Verification items for this drawing (mm, ordinates from the low corner). Give positions to 0.01 mm unless a question says otherwise; leave off trailing zeros. Write each loop counter-clockwise with the first axis right and the second up, starting at its lowest first coordinate (ties: lowest second). Pieces come first, ordered by that corner, then holes. Notation, with made-up numbers: (48.5, 36) -> (69.5, 36) arc R6 ccw to (69.5, 43) -> close; hole circle Ø5 at (28.25, 74.5). An arc over 180 degrees is marked (long way). Answer as a JSON object with one key per item and string values.
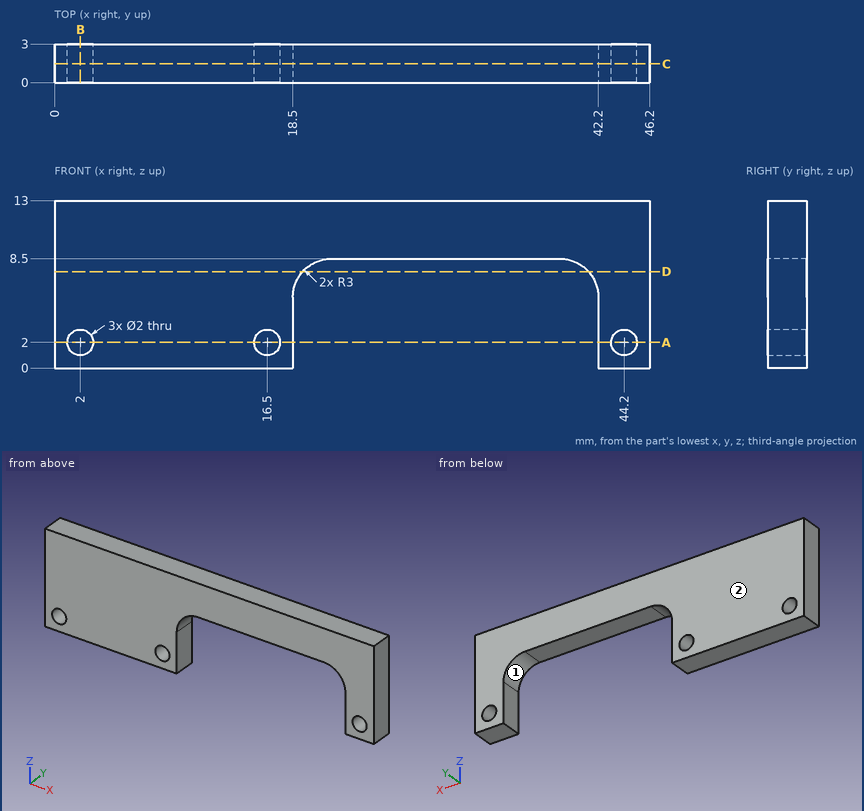
1. Sectioned sample at D-D, the plane z = 7.5. Enter the section's corners in (x, y), plus the area to 3 significant figures.
Determined:
{"outline": "(0, 0) -> (19.26, 0) -> (19.26, 3) -> (0, 3) -> close; (41.44, 0) -> (46.2, 0) -> (46.2, 3) -> (41.44, 3) -> close", "area": "72.1 mm^2"}
2. Sectioned sample at B-B, the plane x = 2. Enter the section's corners in (y, z).
Determined:
{"outline": "(0, 0) -> (3, 0) -> (3, 1) -> (0, 1) -> close; (0, 3) -> (3, 3) -> (3, 13) -> (0, 13) -> close"}
3. Scan lines: L1, parallel to X at y = 0.65, z = 2; L2, parallel to X at y = 1.7, z = 4; L3, parallel to X at y = 0.5, z = 7. Record each from-to range of solid material in increasing order. Write a range as [from, to].
Determined:
{"L1": "[0, 1], [3, 15.5], [17.5, 18.5], [42.2, 43.2], [45.2, 46.2]", "L2": "[0, 18.5], [42.2, 46.2]", "L3": "[0, 18.9], [41.8, 46.2]"}
4. Sectioned sample at C-C, the plane y = 1.45. Enter the section's corners in (x, z), plus the area to 3 significant figures.
Determined:
{"outline": "(0, 0) -> (18.5, 0) -> (18.5, 5.5) arc R3 cw to (21.5, 8.5) -> (39.2, 8.5) arc R3 cw to (42.2, 5.5) -> (42.2, 0) -> (46.2, 0) -> (46.2, 13) -> (0, 13) -> close; hole circle Ø2 at (2, 2); hole circle Ø2 at (16.5, 2); hole circle Ø2 at (44.2, 2)", "area": "394 mm^2"}
5. Mould release check, pull along X, two halves, no side actions. Record for the marked faces 1 and 2: released by +X, released by -X, zero draft, split by the parting line, or undercut.
Determined:
{"face 1": "undercut", "face 2": "zero draft"}
6. Go/stop test with a flat-tipped pin: P1, Ø1.5, axis at x = 32, y = 1.5, coming from the -Z side. Record where the tip stops, or that it passes through.
Determined:
{"P1": "z = 8.5"}
7. Sectioned sample at A-A, the plane z = 2. Enter the section's corners in (x, y), plus the area to 3 significant figures.
Determined:
{"outline": "(0, 0) -> (1, 0) -> (1, 3) -> (0, 3) -> close; (3, 0) -> (15.5, 0) -> (15.5, 3) -> (3, 3) -> close; (17.5, 0) -> (18.5, 0) -> (18.5, 3) -> (17.5, 3) -> close; (42.2, 0) -> (43.2, 0) -> (43.2, 3) -> (42.2, 3) -> close; (45.2, 0) -> (46.2, 0) -> (46.2, 3) -> (45.2, 3) -> close", "area": "49.5 mm^2"}
